Design review of the part built by this model. Coordinates are the model's own, in mm. Face numbers are marked on the shaded views. A direction names the side the tool comes from. Round coordinates to 2 decimals unless told otherwise and drop trailing zeros. Write each loop counter-clockwise with the first axis right and the second up, starting at its lowest first coordinate (ties: lowest second). Pieces come first, ordered by that corner, then holes. Notation, with made-up numbers: M 20,80 L 40,80 A22 ccw 40,86 Z; hole C 86.5,79.5 d2. An arc over 180 degrees is marked long. One line per question, with ' | ' between items. Start each with the question number.
Item 1: Insertion check: pin 1 Ø3 at (x, z) = (-6, -3.5) entering from +Y; pin 2 Ø6 at (y, z) = (-12.5, -7.5) entering from -X; pin 3 Ø8 at (x, y) = (-0.5, 12) entering from +Z; pin 4 Ø1 at (y, z) = (15, 10) entering from +X. Each pin has a flat end and moves straight along its axis. Give the tip position at first contact, or say it passes through.
Item 2: Add section C-C, the plane x = 8.5. State the section outline as (y, z) points.
Item 3: Add section B-B, the plane x = 21.5. Give the number of separate pieces and of enclosed holes in the cut face, and give its area (3 significant figures).
Item 4: Machinability: for the marked faces 1 and 2, which of the approach directions +Z, -Z, +X, -X, +Y, -Y give a long, thin tool a straight path to every point of the face, cutting with its end or side? Answer none if there is none.
Item 5: Add section A-A, the plane x = -10. State the section outline as (y, z) points.
Item 6: For L1, parallel to Y at x = 27, z = 5; L2, parallel to Y at x = 12, z = 6; L3, parallel to Z at x = 29, y = 3, list the stretches that pass through material, from the lowest coordinate up.
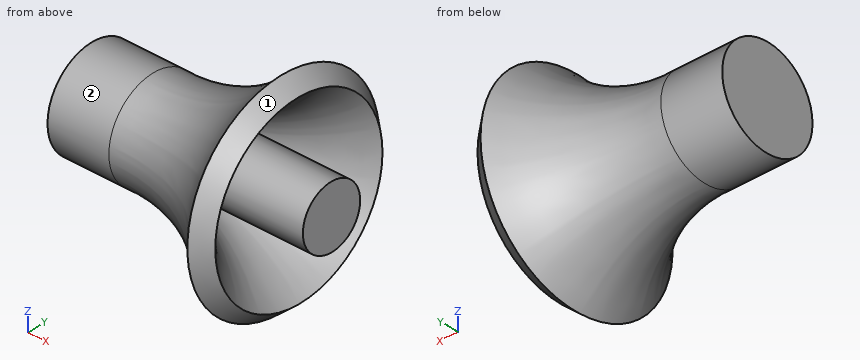
```python
from build123d import *

# Parameters (mm, degrees)
F1_FACE_R = 11.855998
F2_DEPTH  = 15


with BuildPart() as f1:
    # F0 (on Top) → F1 (revolve)
    with BuildSketch(Plane.XY):
        with BuildLine():
            Line((0, 6.848679), (0, 0))
            Line((0, 0), (43.378383, 0))
            Line((43.378383, 0), (43.378383, 2.531673))
            Line((43.378383, 2.531673), (43.378383, 7.531673))
            Line((43.378383, 7.531673), (10.226769, 7.527062))
            ThreePointArc((10.226769, 7.527062), (24.044458, 12.602389), (35.404081, 21.964357))
            Line((35.404081, 21.964357), (31.621624, 25.234375))
            ThreePointArc((31.621624, 25.234375), (17.368897, 14.862439), (0, 11.855998))
            Line((0, 11.855998), (0, 6.848679))
        make_face()
    revolve(axis=Axis((21.689191, 0, 0), (-1, 0, 0)))

    # F1_face (on face) → F2 (join)
    with BuildSketch(Plane(origin=(0, 0, 0), x_dir=(0, -1, 0), z_dir=(-1, 0, 0))):
        Circle(F1_FACE_R)
    extrude(amount=F2_DEPTH)


solid = f1.part
```
Computed values:
1) pin 1: stops at y = 11.69 | pin 2: stops at x = -15 | pin 3: stops at z = 8.75 | pin 4: stops at x = 32.09
2) outline: C 0,0 d24.6
3) separate pieces: 2 | enclosed holes: 1 | area: 678 mm^2
4) face 1: +X | face 2: -X
5) outline: C 0,0 d23.71
6) L1: y = -20.1 to -13.57, -5.63 to 5.63, 13.57 to 20.1 | L2: y = -11.58 to -5.13, -4.55 to 4.55, 5.13 to 11.58 | L3: z = -22.28 to -15.63, -6.91 to 6.91, 15.63 to 22.28
